Can you work these out from the model? Positions are in its coordinate system, mm. Give positions to 0.01 mm unless a question says otherwise; leave off trailing zeros. Write each loop counter-clockwise with the first axis right and the second up, starting at its lowest first coordinate (ties: lowest second). Pieces come first, ordered by that corner, then holes.
1. Suppose I cut it at B-B (y = 58.5). Please give me the cut outline in (x, z), and give its area (3 significant figures).
2. Suppose I cut it at A-A (x = 15.5). Please give me the cut outline in (y, z).
3. If I drill on probe 1 along X at (y, z) = (60, 6.75); probe 2 along X at (y, z) = (29, 1.25); probe 3 along Z at (x, y) = (12.5, 60.5), over which ranges is the centre line in solid material (lowest first)?
4. I'm going to push a flat-ended pin straight in: pin 1 (3 mm diameter, centred on x = -17, y = 32, fed in from +Z). Where does the tip first touch, or does it pass through?
5. Suppose I cut it at C-C (z = 1.5). Please give me the cut outline in (x, y).
```python
from build123d import *

# Parameters (mm, degrees)
SKETCH_1_W          = 50
SKETCH_1_H          = 140
EXTRUDE_1_DEPTH     = 8
CUT_EXTRUDE_2_DEPTH = 8
CUT_EXTRUDE_3_DEPTH = 3


with BuildPart() as part:
    # 草圖1 → 填料-伸長1 (new body)
    with BuildSketch(Plane.XY):
        Rectangle(SKETCH_1_W, SKETCH_1_H)
    extrude(amount=EXTRUDE_1_DEPTH)

    # 草圖8 → 除料-伸長2 (cut)
    with BuildSketch(Plane.XY.offset(8)):
        with BuildLine():
            Line((-13.85, 65), (-13.85, 55))
            ThreePointArc((-13.85, 55), (-15.5, 53.35), (-17.15, 55))
            Line((-17.15, 55), (-17.15, 65))
            ThreePointArc((-17.15, 65), (-15.5, 66.65), (-13.85, 65))
        make_face()
        with BuildLine():
            Line((13.85, 65), (13.85, 55))
            ThreePointArc((13.85, 55), (15.5, 53.35), (17.15, 55))
            Line((17.15, 55), (17.15, 65))
            ThreePointArc((17.15, 65), (15.5, 66.65), (13.85, 65))
        make_face()
        with BuildLine():
            Line((13.85, 34), (13.85, 24))
            ThreePointArc((13.85, 24), (15.5, 22.35), (17.15, 24))
            Line((17.15, 24), (17.15, 34))
            ThreePointArc((17.15, 34), (15.5, 35.65), (13.85, 34))
        make_face()
        with BuildLine():
            Line((-17.15, 34), (-17.15, 24))
            ThreePointArc((-17.15, 24), (-15.5, 22.35), (-13.85, 24))
            Line((-13.85, 24), (-13.85, 34))
            ThreePointArc((-13.85, 34), (-15.5, 35.65), (-17.15, 34))
        make_face()
    extrude(amount=-CUT_EXTRUDE_2_DEPTH, mode=Mode.SUBTRACT)

    # 草圖9 → 除料-伸長3 (cut)
    with BuildSketch(Plane.XY.offset(8)):
        with BuildLine():
            Line((-12.25, 65), (-12.25, 55))
            ThreePointArc((-12.25, 55), (-15.5, 51.75), (-18.75, 55))
            Line((-18.75, 55), (-18.75, 65))
            ThreePointArc((-18.75, 65), (-15.5, 68.25), (-12.25, 65))
        make_face()
        with BuildLine():
            Line((12.25, 65), (12.25, 55))
            ThreePointArc((12.25, 55), (15.5, 51.75), (18.75, 55))
            Line((18.75, 55), (18.75, 65))
            ThreePointArc((18.75, 65), (15.5, 68.25), (12.25, 65))
        make_face()
        with BuildLine():
            Line((12.25, 34), (12.25, 24))
            ThreePointArc((12.25, 24), (15.5, 20.75), (18.75, 24))
            Line((18.75, 24), (18.75, 34))
            ThreePointArc((18.75, 34), (15.5, 37.25), (12.25, 34))
        make_face()
        with BuildLine():
            Line((-18.75, 34), (-18.75, 24))
            ThreePointArc((-18.75, 24), (-15.5, 20.75), (-12.25, 24))
            Line((-12.25, 24), (-12.25, 34))
            ThreePointArc((-12.25, 34), (-15.5, 37.25), (-18.75, 34))
        make_face()
    extrude(amount=-CUT_EXTRUDE_3_DEPTH, mode=Mode.SUBTRACT)


solid = part.part
```
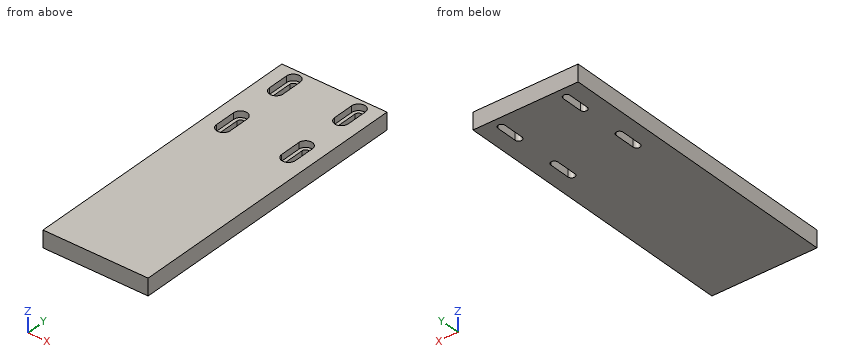
Checks:
1. outline: (-25, 0) - (-17.15, 0) - (-17.15, 5) - (-18.75, 5) - (-18.75, 8) - (-25, 8) - close; (-13.85, 0) - (13.85, 0) - (13.85, 5) - (12.25, 5) - (12.25, 8) - (-12.25, 8) - (-12.25, 5) - (-13.85, 5) - close; (17.15, 0) - (25, 0) - (25, 8) - (18.75, 8) - (18.75, 5) - (17.15, 5) - close
1. area: 328 mm2
2. outline: (-70, 0) - (22.35, 0) - (22.35, 5) - (20.75, 5) - (20.75, 8) - (-70, 8) - close; (35.65, 0) - (53.35, 0) - (53.35, 5) - (51.75, 5) - (51.75, 8) - (37.25, 8) - (37.25, 5) - (35.65, 5) - close; (66.65, 0) - (70, 0) - (70, 8) - (68.25, 8) - (68.25, 5) - (66.65, 5) - close
3. probe 1: x = -25 to -18.75, -12.25 to 12.25, 18.75 to 25
3. probe 2: x = -25 to -17.15, -13.85 to 13.85, 17.15 to 25
3. probe 3: z = 0 to 5
4. pin 1: stops at z = 5
5. outline: (-25, -70) - (25, -70) - (25, 70) - (-25, 70) - close; hole (-17.15, 24) arc R1.65 ccw to (-13.85, 24) - (-13.85, 34) arc R1.65 ccw to (-17.15, 34) - close; hole (-17.15, 55) arc R1.65 ccw to (-13.85, 55) - (-13.85, 65) arc R1.65 ccw to (-17.15, 65) - close; hole (13.85, 24) arc R1.65 ccw to (17.15, 24) - (17.15, 34) arc R1.65 ccw to (13.85, 34) - close; hole (13.85, 55) arc R1.65 ccw to (17.15, 55) - (17.15, 65) arc R1.65 ccw to (13.85, 65) - close
